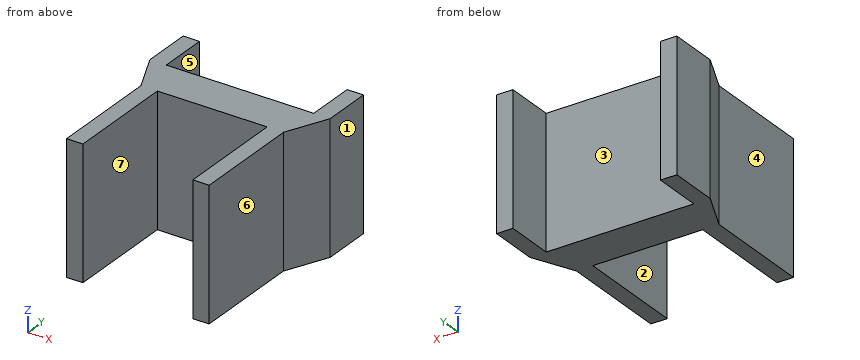
```python
from build123d import *

# Parameters (mm, degrees)
CROQUIS1_W              = 2
CROQUIS1_H              = 13.4
CROQUIS1_H_2            = 6
SALIENTE_EXTRUIR1_DEPTH = 16


with BuildPart() as part:
    # Croquis1 → Saliente-Extruir1 (new body)
    with BuildSketch(Plane.XY):
        with Locations((-1, -6.7)):
            Rectangle(CROQUIS1_W, CROQUIS1_H)
        Polygon((15.4, 5), (6.7, 5), (-2, 5), (-2, 0), (0, 0), (13.4, 0), (15.4, 0), align=None)
        with Locations((14.4, -6.7)):
            Rectangle(CROQUIS1_W, CROQUIS1_H)
        Polygon((15.7, 5), (15.4, 5), (15.4, 0), (17.7, 5), align=None)
        with Locations((16.7, 8)):
            Rectangle(CROQUIS1_W, CROQUIS1_H_2)
        Polygon((-2, 0), (-2, 5), (-2.3, 5), (-4.3, 5), align=None)
        with Locations((-3.3, 8)):
            Rectangle(CROQUIS1_W, CROQUIS1_H_2)
    extrude(amount=SALIENTE_EXTRUIR1_DEPTH)


solid = part.part
```
Could you check a few things on this model? Use its own coordinates, in mm. Face numbers are marked on the shaded views. A direction names the side the tool comes from. Coordinates: 2 decimals unless noted, no trailing zeros. Write each loop counter-clockwise with the first axis right and the second up, starting at its lowest first coordinate (ties: lowest second). Pieces come first, ordered by that corner, then holes. Notation, with made-up numbers: (2, 14) -> (25, 14) arc R36 cw to (25, 53) -> close; hole circle Ø5 at (68, 16.5). An arc over 180 degrees is marked (long way). Write item = value, one per line. Start each with the question number.
(1) I want a section at C-C (x = 4). Please give me the cut outline in (y, z).
(2) I need wall thicknesses on line 1 (X direction, y = -6.5, z = 5.25); line 2 (X direction, y = 9.25, z = 11); line 3 (Y direction, x = 6.75, z = 11.5). Which ranges of each line are inside material? Lowest first, please. Write a range as [from, to].
(3) Will these pins go through, and if not, where does the flat tip stop? pin 1 (6.5 mm diameter, centred on y = -10, z = 10.5, fed in from +X); pin 2 (2 mm diameter, centred on x = 14.5, z = 9, fed in from +Y); pin 3 (6.5 mm diameter, centred on y = -10, z = 4.5, fed in from -X).
(4) Which directions (+Z, -Z, +X, -X, +Y, -Y) give clear straight access to the entire face, cutting with the end or side of a thin tool? Please do the marked faces 5, 6 and 7.
(5) I want a section at B-B (z = 7.5). Please give me the cut outline in (x, y), plus the area to 3 significant figures.
(6) I want a section at A-A (y = -5). Please give me the cut outline in (x, z), plus the area to 3 significant figures.
(7) I want a section at D-D (y = 4.5). Please give me the cut outline in (x, z).
(8) We'd pull the mould along X, two halves only. Please class the marked faces 1, 2, 3 and 4: released by +X, released by -X, zero draft, split by the parting line, or undercut.
Result set:
q1.outline = (0, 0) -> (5, 0) -> (5, 16) -> (0, 16) -> close
q2.line_1 = [-2, 0], [13.4, 15.4]
q2.line_2 = [-4.3, -2.3], [15.7, 17.7]
q2.line_3 = [0, 5]
q3.pin_1 = 15.4
q3.pin_2 = 5
q3.pin_3 = -2
q4.face_5 = +Z, -Z, +Y
q4.face_6 = +Z, -Z, +X, -Y
q4.face_7 = +Z, -Z, -Y
q5.outline = (-4.3, 5) -> (-2, 0) -> (-2, -13.4) -> (0, -13.4) -> (0, 0) -> (13.4, 0) -> (13.4, -13.4) -> (15.4, -13.4) -> (15.4, 0) -> (17.7, 5) -> (17.7, 11) -> (15.7, 11) -> (15.7, 5) -> (-2.3, 5) -> (-2.3, 11) -> (-4.3, 11) -> close
q5.area = 176 mm2
q6.outline = (-2, 0) -> (0, 0) -> (0, 16) -> (-2, 16) -> close; (13.4, 0) -> (15.4, 0) -> (15.4, 16) -> (13.4, 16) -> close
q6.area = 64.0 mm2
q7.outline = (-4.07, 0) -> (17.47, 0) -> (17.47, 16) -> (-4.07, 16) -> close
q8.face_1 = released by +X
q8.face_2 = undercut
q8.face_3 = undercut
q8.face_4 = released by -X
